Can you work these out from the model? Positions are in its coordinate system, mm. A direction names the side the tool comes from. Round coordinates to 2 decimals unless told otherwise and drop trailing zeros. Loops run counter-clockwise (first coordinate to the right, second up) from the corner with the lowest first, then second, coordinate; pieces in that order, holes last.
```python
from build123d import *

# Parameters (mm, degrees)
CROQUIS1_R              = 22.5
SALIENTE_EXTRUIR1_DEPTH = 15
CROQUIS2_R              = 15
SALIENTE_EXTRUIR2_DEPTH = 102
CROQUIS4_R              = 2.957727645
CORTAR_EXTRUIR1_DEPTH   = 48.5


with BuildPart() as part:
    # Croquis1 → Saliente-Extruir1 (new body)
    with BuildSketch(Plane(origin=(0, 0, 0), x_dir=(1, 0, 0), z_dir=(0, 1, 0))):
        with Locations(Location((0, 0, 0), (0, 0, 270))):
            Circle(CROQUIS1_R)
    extrude(amount=-SALIENTE_EXTRUIR1_DEPTH)

    # Croquis2 → Saliente-Extruir2 (add)
    with BuildSketch(Plane.XZ.offset(15)):
        with Locations(Location((0, 0, 0), (0, 0, 270))):
            Circle(CROQUIS2_R)
    extrude(amount=SALIENTE_EXTRUIR2_DEPTH)

    # Croquis4 → Cortar-Extruir1 (cut, symmetric)
    with BuildSketch(Plane.XY):
        with Locations(Location((0, -102, 0), (0, 0, 269.999999959))):
            Circle(CROQUIS4_R)
    extrude(amount=CORTAR_EXTRUIR1_DEPTH, both=True, mode=Mode.SUBTRACT)


solid = part.part
```
(1) Suppose I cut it at C-C (y = -102). Write out the boundary of the cut face in (x, z).
(2) If I drill on line 1 (Y direction, x = 0, z = -3); line 2 (Y direction, x = -15, z = -7.5); line 3 (X direction, y = -102, z = 0), over which ranges is the centre line in solid material (lowest first)?
(3) For pin 1 (3 mm diameter, centred on x = -17.5, z = -10.5, fed in from -Y); pin 2 (12 mm diameter, centred on y = -36, z = -12.5, fed in from +X); pin 3 (4 mm diameter, centred on y = -85.5, z = -7, fed in from -X), each with a flat end and sliding along its axis, tell me the tip position at first contact or that it passes through.
(4) Suppose I cut it at D-D (x = 9). Write out the boundary of the cut face in (y, z).
(5) Suppose I cut it at A-A (z = 0). Write out the boundary of the cut face in (x, y), then the cut area to 3 significant figures.
(6) Suppose I cut it at B-B (x = 0). Write out the boundary of the cut face in (y, z).
(7) Which directions (+Z, -Z, +X, -X, +Y, -Y) give clear straight access to the entire face, cutting with the end or side of a thin tool? Please do faces 5 (the cylindrical face through (-5.745, -65.286, -13.856)), 6 (the flat face through (0, -117, 0)).
(8) We'd pull the mould along Y, two halves only. Please class faces 1 (the flat face through (0, 0, 0)), 2 (the cylindrical face through (0.13, -99.045, 0.212)), 3 (the cylindrical face through (-8.618, -7.395, 20.784)), 4 (the flat face through (-5, -15, 15)): released by +Y, released by -Y, zero draft, split by the parting line, or undercut.
Check result:
1. outline: (-2.96, -14.71) - (-2.96, 14.71) arc R15 ccw to start; (2.96, -14.71) arc R15 ccw to (2.96, 14.71) - close
2. line 1: y = -117 to -104.96, -99.04 to 0
2. line 2: y = -15 to 0
2. line 3: x = -15 to -2.96, 2.96 to 15
3. pin 1: stops at y = -15
3. pin 2: stops at x = 13.52
3. pin 3: stops at x = -14.14
4. outline: (-117, -12) - (-15, -12) - (-15, -20.62) - (0, -20.62) - (0, 20.62) - (-15, 20.62) - (-15, 12) - (-117, 12) - close
5. outline: (-22.5, -15) - (-15, -15) - (-15, -117) - (15, -117) - (15, -15) - (22.5, -15) - (22.5, 0) - (-22.5, 0) - close; hole circle Ø5.92 at (0, -102)
5. area: 3,710 mm2
6. outline: (-117, -15) - (-104.96, -15) - (-104.96, 15) - (-117, 15) - close; (-99.04, -15) - (-15, -15) - (-15, -22.5) - (0, -22.5) - (0, 22.5) - (-15, 22.5) - (-15, 15) - (-99.04, 15) - close
7. face 5: -Y
7. face 6: +Z, -Z, +X, -X, -Y
8. face 1: released by +Y
8. face 2: undercut
8. face 3: zero draft
8. face 4: released by -Y
